Source: CAD feature listing. Evaluate the final solid. Frame: model axes, mm. Face numbers are marked on the shaded views. A direction names the side the tool comes from. Round coordinates to 2 decimals unless told otherwise and drop trailing zeros. Loops run counter-clockwise (first coordinate to the right, second up) from the corner with the lowest first, then second, coordinate; pieces in that order, holes last. Notation, with made-up numbers: (-9, 40) - (-3, 40) arc R20 ccw to (-3, 76) - close; hole circle Ø8 at (56, 47.25). An arc over 180 degrees is marked (long way). Write item = value, one per line. Start each with the question number.
from build123d import *

# Parameters (mm, degrees)
EXTRUDE_1_DEPTH          = 11
CUT_EXTRUDE_1_DEPTH      = 50.648766349
CUT_EXTRUDE_1_DEPTH_BACK = 50.648766349
SKETCH_3_R               = 1.5
SKETCH_4_R               = 3
CUT_EXTRUDE_2_DEPTH      = 3


with BuildPart() as part:
    # 草图2 → 凸台-拉伸1 (new body)
    with BuildSketch(Plane.XY):
        Polygon((0, 30), (0, 0), (38, 0), (38, 30), (36, 30), (36, 2), (2, 2), (2, 30), align=None)
    extrude(amount=EXTRUDE_1_DEPTH)

    # 草图3 → 切除-拉伸1 (cut, two sides: drawn at the far end of the back side and taken through both)
    with BuildSketch(Plane.ZY.offset(-CUT_EXTRUDE_1_DEPTH_BACK)):
        with Locations((5.5, 27)):
            Circle(SKETCH_3_R)
    extrude(amount=CUT_EXTRUDE_1_DEPTH + CUT_EXTRUDE_1_DEPTH_BACK, mode=Mode.SUBTRACT)

    # 草图4 → 切除-拉伸2 (cut)
    with BuildSketch(Plane.XZ):
        with Locations(Location((19, 5.5, 0), (0, 0, 270))):
            Circle(SKETCH_4_R)
        with BuildLine():
            Line((26.5, 7), (31.5, 7))
            ThreePointArc((31.5, 7), (33, 5.5), (31.5, 4))
            Line((31.5, 4), (26.5, 4))
            ThreePointArc((26.5, 4), (25, 5.5), (26.5, 7))
        make_face()
        with BuildLine():
            Line((6.5, 7), (11.5, 7))
            ThreePointArc((11.5, 7), (13, 5.5), (11.5, 4))
            Line((11.5, 4), (6.5, 4))
            ThreePointArc((6.5, 4), (5, 5.5), (6.5, 7))
        make_face()
    extrude(amount=-CUT_EXTRUDE_2_DEPTH, mode=Mode.SUBTRACT)


solid = part.part
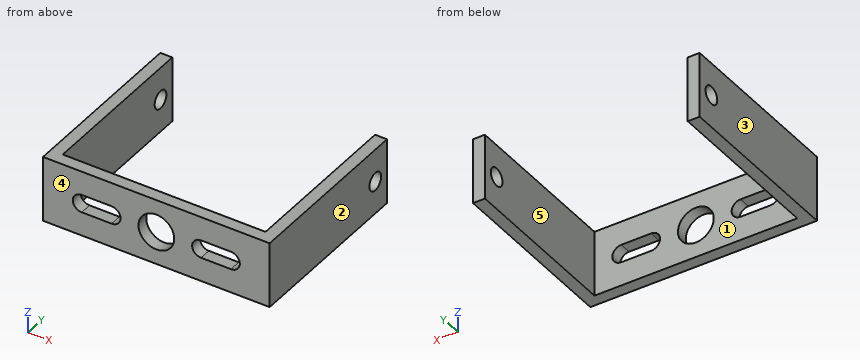
(1) Access query for the marked faces 4 and 5. Directions: +Z, -Z, +X, -X, +Y, -Y. A direction counts if a zero-diameter tool reaches every point of the face in a straight line with its end or side. Return the directions, or none.
(2) Mould query, pull axis X, two halves, no side actions, for the marked faces 1, 2 and 3. Classes: +X half, -X half, draft (parallel to the pull), parting line (faces both ways), or undercut.
(3) Cut plane A-A (z = 5.5). Output: boundary loops of the cut face in (x, y), and give its area (3 significant figures).
(4) Pin query (flat end, axial travel): P1, Ø0.6, axis at x = 29, y = 1, coming from the -Z side; P2, Ø2.5, axis at y = 27, z = 5.5, coming from the -X side; P3, Ø3.5, axis at x = 26.5, z = 7.5, coming from the +Y side. Return the tip coordinate at first contact, or that it passes through.
(5) Cut plane C-C (x = 19). Output: boundary loops of the cut face in (y, z).
(6) Cut plane B-B (y = 4.5). Output: boundary loops of the cut face in (x, z).
(7) Cut plane D-D (y = 27). Output: boundary loops of the cut face in (x, z), and give its area (3 significant figures).
(8) Material intervals for line 1 along X through (y, z) = (1.2, 5.5); line 2 along Y through (x, z) = (0.9, 5.5); line 3 along X through (y, z) = (26.5, 4), sorted ascending. Write a range as from..to.
Solution:
q1.face_4 = +Z, -Z, +X, -X, -Y
q1.face_5 = +Z, -Z, +Y
q2.face_1 = undercut
q2.face_2 = +X half
q2.face_3 = -X half
q3.outline = (0, 0) - (5, 0) - (5, 2) - (2, 2) - (2, 25.5) - (0, 25.5) - close; (0, 28.5) - (2, 28.5) - (2, 30) - (0, 30) - close; (13, 0) - (16, 0) - (16, 2) - (13, 2) - close; (22, 0) - (25, 0) - (25, 2) - (22, 2) - close; (33, 0) - (38, 0) - (38, 25.5) - (36, 25.5) - (36, 2) - (33, 2) - close; (36, 28.5) - (38, 28.5) - (38, 30) - (36, 30) - close
q3.area = 132 mm^2
q4.P1 = 0
q4.P2 = through
q4.P3 = 2
q5.outline = (0, 0) - (2, 0) - (2, 2.5) - (0, 2.5) - close; (0, 8.5) - (2, 8.5) - (2, 11) - (0, 11) - close
q6.outline = (0, 0) - (2, 0) - (2, 11) - (0, 11) - close; (36, 0) - (38, 0) - (38, 11) - (36, 11) - close
q7.outline = (0, 0) - (2, 0) - (2, 4) - (0, 4) - close; (0, 7) - (2, 7) - (2, 11) - (0, 11) - close; (36, 0) - (38, 0) - (38, 4) - (36, 4) - close; (36, 7) - (38, 7) - (38, 11) - (36, 11) - close
q7.area = 32.0 mm^2
q8.line_1 = 0..5, 13..16, 22..25, 33..38
q8.line_2 = 0..25.5, 28.5..30
q8.line_3 = 0..2, 36..38
